```python
from build123d import *

# Parameters (mm, degrees)
F0_R     = 2.25
F1_DEPTH = 3
F2_SIZE  = 10
F3_R     = 3.25
F4_DEPTH = 1


with BuildPart() as f1:
    # F0 (on Front) → F1 (new body)
    with BuildSketch(Plane.XZ):
        Polygon((115, 65), (-115, 65), (-115, -65), (-65, -65), (-65, -25), (0, -25), (65, -25), (65, -65), (115, -65), align=None)
        with Locations((-83, -35)):
            Circle(F0_R, mode=Mode.SUBTRACT)
        with Locations((83, -35)):
            Circle(F0_R, mode=Mode.SUBTRACT)
        with Locations((-83, 0)):
            Circle(F0_R, mode=Mode.SUBTRACT)
        with Locations((0, 5)):
            Circle(F0_R, mode=Mode.SUBTRACT)
        with Locations((0, 20)):
            Circle(F0_R, mode=Mode.SUBTRACT)
        with Locations((83, 0)):
            Circle(F0_R, mode=Mode.SUBTRACT)
    extrude(amount=F1_DEPTH)

    # F2
    f2_edges = [f1.edges().sort_by_distance(p)[0] for p in [
        (-115, -1.5, 65),
        (115, -1.5, 65),
        (115, -1.5, -65),
        (-115, -1.5, -65),
    ]]
    chamfer(f2_edges, length=F2_SIZE)

    # F3 (on face) → F4 (cut)
    with BuildSketch(Plane.XZ.offset(3)):
        with Locations((-83, 0)):
            Circle(F3_R)
        with Locations((-83, -35)):
            Circle(F3_R)
        with Locations((0, 20)):
            Circle(F3_R)
        with Locations((0, 5)):
            Circle(F3_R)
        with Locations((83, 0)):
            Circle(F3_R)
        with Locations((83, -35)):
            Circle(F3_R)
    extrude(amount=-F4_DEPTH, mode=Mode.SUBTRACT)


solid = f1.part
```
For this review, take the finished solid that the model builds, in its own axes (mm). A direction names the side the tool comes from. Give positions to 0.01 mm unless a question says otherwise; leave off trailing zeros. Order: outer loops, then holes, each group sorted by start corner. A loop starts at its lowest first (then second) coordinate and runs counter-clockwise, first axis right, second up.
1) For faces 4 (the face through (-0.705, -2.507, 16.827)), 5 (the face through (-80.92, -0.99, -0.86)), list the 3-axis set-ups (+Z, -Z, +X, -X, +Y, -Y) from which the entire face can be reached by the end or side of a thin tool; tool diameter is ignored.
2) The part is to be moulded in two halves that separate along Z. For faces 1 (the face through (-2, -3, 15)), 2 (the face through (-86.247, -2.507, 0.143)), 3 (the face through (-110, -1, 60)), say which applies: released by +Z, released by -Z, zero draft, split by the parting line, or undercut.
3) Wall thickness on line 1 (X direction, y = -0.5, z = 0); line 2 (X direction, y = -0.75, z = -35); line 3 (Z direction, x = 0, y = -2.6): over which ranges is each line inside the solid? List them lowest first.
4) Take a section at B-B (y = -1.5). Give the boundary of the cut face in (x, z).
5) Take a section at C-C (z = -35). Give the boundary of the cut face in (x, y).
6) Take a section at D-D (x = 0). Give the boundary of the cut face in (y, z), then the cut area to 3 significant figures.
7) Take a section at A-A (x = -83). Give the boundary of the cut face in (y, z), then the cut area to 3 significant figures.
Derived:
1. face 4: -Y
1. face 5: +Y, -Y
2. face 1: zero draft
2. face 2: undercut
2. face 3: released by +Z
3. line 1: x = -115 to -85.25, -80.75 to 80.75, 85.25 to 115
3. line 2: x = -115 to -85.25, -80.75 to -65, 65 to 80.75, 85.25 to 115
3. line 3: z = -25 to 1.75, 8.25 to 16.75, 23.25 to 65
4. outline: (-115, -55) - (-105, -65) - (-65, -65) - (-65, -25) - (65, -25) - (65, -65) - (105, -65) - (115, -55) - (115, 55) - (105, 65) - (-105, 65) - (-115, 55) - close; hole circle Ø4.5 at (-83, -35); hole circle Ø4.5 at (-83, 0); hole circle Ø4.5 at (0, 5); hole circle Ø4.5 at (0, 20); hole circle Ø4.5 at (83, -35); hole circle Ø4.5 at (83, 0)
5. outline: (-115, -3) - (-86.25, -3) - (-86.25, -2) - (-85.25, -2) - (-85.25, 0) - (-115, 0) - close; (-80.75, -2) - (-79.75, -2) - (-79.75, -3) - (-65, -3) - (-65, 0) - (-80.75, 0) - close; (65, -3) - (79.75, -3) - (79.75, -2) - (80.75, -2) - (80.75, 0) - (65, 0) - close; (85.25, -2) - (86.25, -2) - (86.25, -3) - (115, -3) - (115, 0) - (85.25, 0) - close
6. outline: (-3, -25) - (0, -25) - (0, 2.75) - (-2, 2.75) - (-2, 1.75) - (-3, 1.75) - close; (-3, 8.25) - (-2, 8.25) - (-2, 7.25) - (0, 7.25) - (0, 17.75) - (-2, 17.75) - (-2, 16.75) - (-3, 16.75) - close; (-3, 23.25) - (-2, 23.25) - (-2, 22.25) - (0, 22.25) - (0, 65) - (-3, 65) - close
6. area: 239 mm2
7. outline: (-3, -65) - (0, -65) - (0, -37.25) - (-2, -37.25) - (-2, -38.25) - (-3, -38.25) - close; (-3, -31.75) - (-2, -31.75) - (-2, -32.75) - (0, -32.75) - (0, -2.25) - (-2, -2.25) - (-2, -3.25) - (-3, -3.25) - close; (-3, 3.25) - (-2, 3.25) - (-2, 2.25) - (0, 2.25) - (0, 65) - (-3, 65) - close
7. area: 359 mm2
